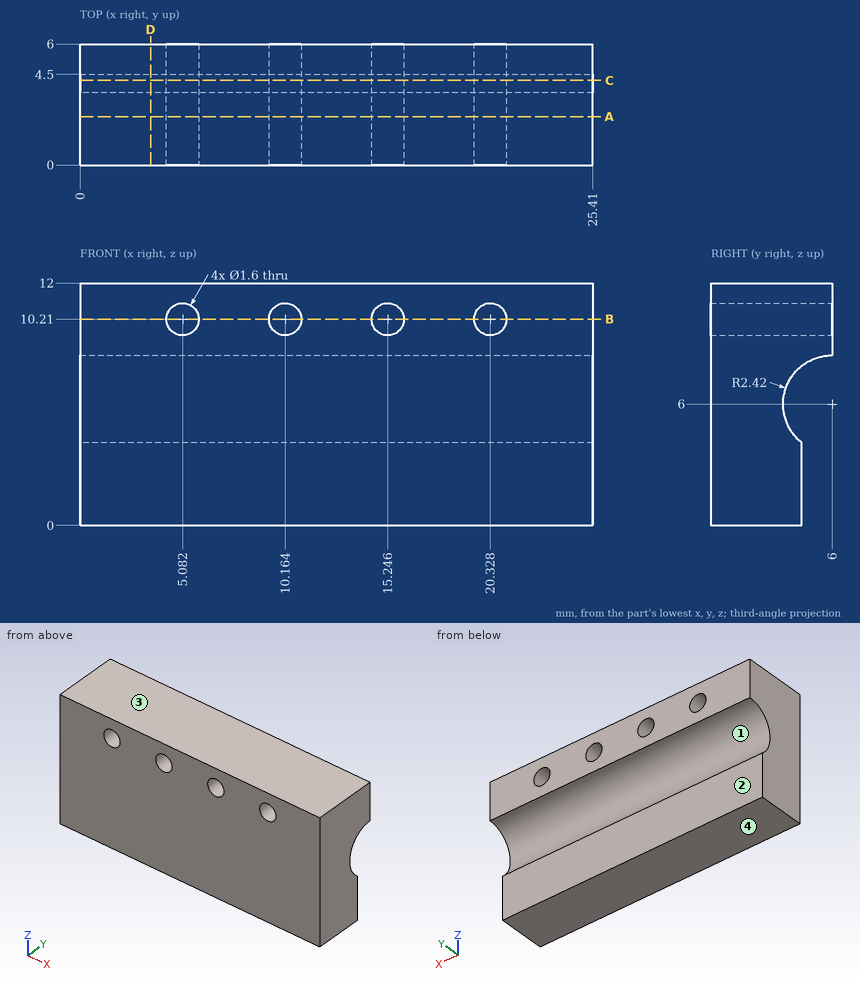
Design review of the part shown in the three views and the two pictorial views. Dimensions are in mm from the part's minimum x, y and z. Round coordinates to 2 decimals unless told otherwise and drop trailing zeros. Order: outer loops, then holes, each group sorted by start corner. A loop starts at its lowest first (then second) coordinate and runs counter-clockwise, first axis right, second up.
(1) Take a section at A-A, the plane y = 2.4. State the section outline as (x, z) points.
Working result:
outline: (0, 0) - (25.41, 0) - (25.41, 12) - (0, 12) - close; hole circle Ø1.6 at (5.08, 10.21); hole circle Ø1.6 at (10.16, 10.21); hole circle Ø1.6 at (15.25, 10.21); hole circle Ø1.6 at (20.33, 10.21)
(2) Take a section at B-B, the plane z = 10.21. State the section outline as (x, y) points, plus the area to 3 significant figures.
Working result:
outline: (0, 0) - (4.28, 0) - (4.28, 6) - (0, 6) - close; (5.88, 0) - (9.36, 0) - (9.36, 6) - (5.88, 6) - close; (10.96, 0) - (14.45, 0) - (14.45, 6) - (10.96, 6) - close; (16.05, 0) - (19.53, 0) - (19.53, 6) - (16.05, 6) - close; (21.13, 0) - (25.41, 0) - (25.41, 6) - (21.13, 6) - close
area: 114 mm2
(3) Wall thickness on L1, parallel to Y at x = 11.25, z = 2.25; L2, parallel to X at y = 2.65, z = 10; L3, parallel to Y at x = 11.75, z = 6: over which ranges is each line inside the solid? List them lowest first.
Working result:
L1: y = 0 to 4.5
L2: x = 0 to 4.31, 5.85 to 9.39, 10.94 to 14.47, 16.02 to 19.56, 21.1 to 25.41
L3: y = 0 to 3.58
(4) Take a section at D-D, the plane x = 3.5. State the section outline as (y, z) points, plus the area to 3 significant figures.
Working result:
outline: (0, 0) - (4.5, 0) - (4.5, 4.1) arc R2.42 cw to (6, 8.42) - (6, 12) - (0, 12) - close
area: 57.2 mm2
(5) Mouldability with a two-part tool opening along Z and no side actions: class the marked faces 1, 2, 3 and 4 as released by +Z, released by -Z, zero draft, split by the parting line, or undercut.
Working result:
face 1: undercut
face 2: zero draft
face 3: released by +Z
face 4: released by -Z
(6) Take a section at C-C, the plane y = 4.2. State the section outline as (x, z) points, plus the area to 3 significant figures.
Working result:
outline: (0, 0) - (25.41, 0) - (25.41, 4.38) - (0, 4.38) - close; (0, 7.62) - (25.41, 7.62) - (25.41, 12) - (0, 12) - close; hole circle Ø1.6 at (5.08, 10.21); hole circle Ø1.6 at (10.16, 10.21); hole circle Ø1.6 at (15.25, 10.21); hole circle Ø1.6 at (20.33, 10.21)
area: 215 mm2
(7) For P1, Ø2, axis at x = 16, z = 3, coming from the +Y side; P2, Ø1.3, axis at x = 20.328, z = 10.21, coming from the -Y side, all flat-tipped, find the tip position at first contact; note any pin that passes through.
Working result:
P1: stops at y = 4.5
P2: passes through
